```python
from build123d import *

# Parameters (mm, degrees)
SKETCH1_R           = 2.2
BOSS_EXTRUDE1_DEPTH = 3


with BuildPart() as part:
    # Sketch1 → Boss-Extrude1 (new body)
    with BuildSketch(Plane.XY):
        with BuildLine():
            Line((18.258523289, 46.816726382), (0, 0))
            Line((0, 0), (0, -3))
            Line((0, -3), (12, -3))
            Line((12, -3), (12, 0))
            Line((12, 0), (25.254184663, 0))
            Line((25.254184663, 0), (34.158272776, 22.830995159))
            ThreePointArc((34.158272776, 22.830995159), (34.413825591, 23.723428265), (34.5, 24.647721542))
            Line((34.5, 24.647721542), (34.5, 45))
            ThreePointArc((34.5, 45), (33.035533906, 48.535533906), (29.5, 50))
            Line((29.5, 50), (22.916796065, 50))
            ThreePointArc((22.916796065, 50), (20.095770711, 49.128173441), (18.258523289, 46.816726382))
        make_face()
        with Locations((26.208398032, 30)):
            Circle(SKETCH1_R, mode=Mode.SUBTRACT)
        with Locations((26.208398032, 45)):
            Circle(SKETCH1_R, mode=Mode.SUBTRACT)
    extrude(amount=BOSS_EXTRUDE1_DEPTH)


solid = part.part
```
Geometry: final body of the model. Coordinates: model frame, mm. A direction names the side the tool comes from. Round coordinates to 2 decimals unless told otherwise and drop trailing zeros. Order: outer loops, then holes, each group sorted by start corner. A loop starts at its lowest first (then second) coordinate and runs counter-clockwise, first axis right, second up. Notation, with made-up numbers: (3, 87.5) -> (45, 87.5) arc R26 cw to (45, 111.5) -> close; hole circle Ø7 at (68.5, -39). An arc over 180 degrees is marked (long way). Write each question's results on one line, items separated by ' | '.
Q1. Access query for faces 5 (the face through (21, 24, 3)), 6 (the face through (12, -2, 1)). Directions: +Z, -Z, +X, -X, +Y, -Y. A direction counts if a zero-diameter tool reaches every point of the face in a straight line with its end or side. Return the directions, or none.
Response values:
face 5: +Z, +X, -X, +Y, -Y | face 6: +Z, -Z, +X, -Y
Q2. Section query D-D (y = 39). Output: boundary loops of the cut face in (x, z), and give its area (3 significant figures).
Response values:
outline: (15.21, 0) -> (34.5, 0) -> (34.5, 3) -> (15.21, 3) -> close | area: 57.9 mm²
Q3. Section query B-B (z = 2.45). Output: boundary loops of the cut face in (x, y).
Response values:
outline: (0, -3) -> (12, -3) -> (12, 0) -> (25.25, 0) -> (34.16, 22.83) arc R5 ccw to (34.5, 24.65) -> (34.5, 45) arc R5 ccw to (29.5, 50) -> (22.92, 50) arc R5 ccw to (18.26, 46.82) -> (0, 0) -> close; hole circle Ø4.4 at (26.21, 30); hole circle Ø4.4 at (26.21, 45)
Q4. Section query A-A (y = 30). Output: boundary loops of the cut face in (x, z).
Response values:
outline: (11.7, 0) -> (24.01, 0) -> (24.01, 3) -> (11.7, 3) -> close; (28.41, 0) -> (34.5, 0) -> (34.5, 3) -> (28.41, 3) -> close
Q5. Ray query, line 1 along X through (y, z) = (22, 0.95); line 2 along X through (y, z) = (37, 0.9). Return the intervals inside material, ascending.
Response values:
line 1: 8.58 to 33.83 | line 2: 14.43 to 34.5
Q6. Pin query (flat end, axial travel): pin 1 Ø4 at (x, y) = (26.21, 45) entering from -Z. Return the tip coordinate at first contact, or that it passes through.
Response values:
pin 1: through
Q7. Pull-direction query (Y, two-part tool) for faces 1 (the face through (34.5, 35, 1)), 2 (the face through (25.731, 27.852, 1.479)), 3 (the face through (25.731, 42.852, 1.479)), 4 (the face through (19, 0, 1)); classes: released by +Y, released by -Y, zero draft, split by the parting line, or undercut.
Response values:
face 1: zero draft | face 2: undercut | face 3: undercut | face 4: released by -Y
Q8. Section query C-C (x = 26.5). Output: boundary loops of the cut face in (y, z).
Response values:
outline: (3.19, 0) -> (27.82, 0) -> (27.82, 3) -> (3.19, 3) -> close; (32.18, 0) -> (42.82, 0) -> (42.82, 3) -> (32.18, 3) -> close; (47.18, 0) -> (50, 0) -> (50, 3) -> (47.18, 3) -> close
